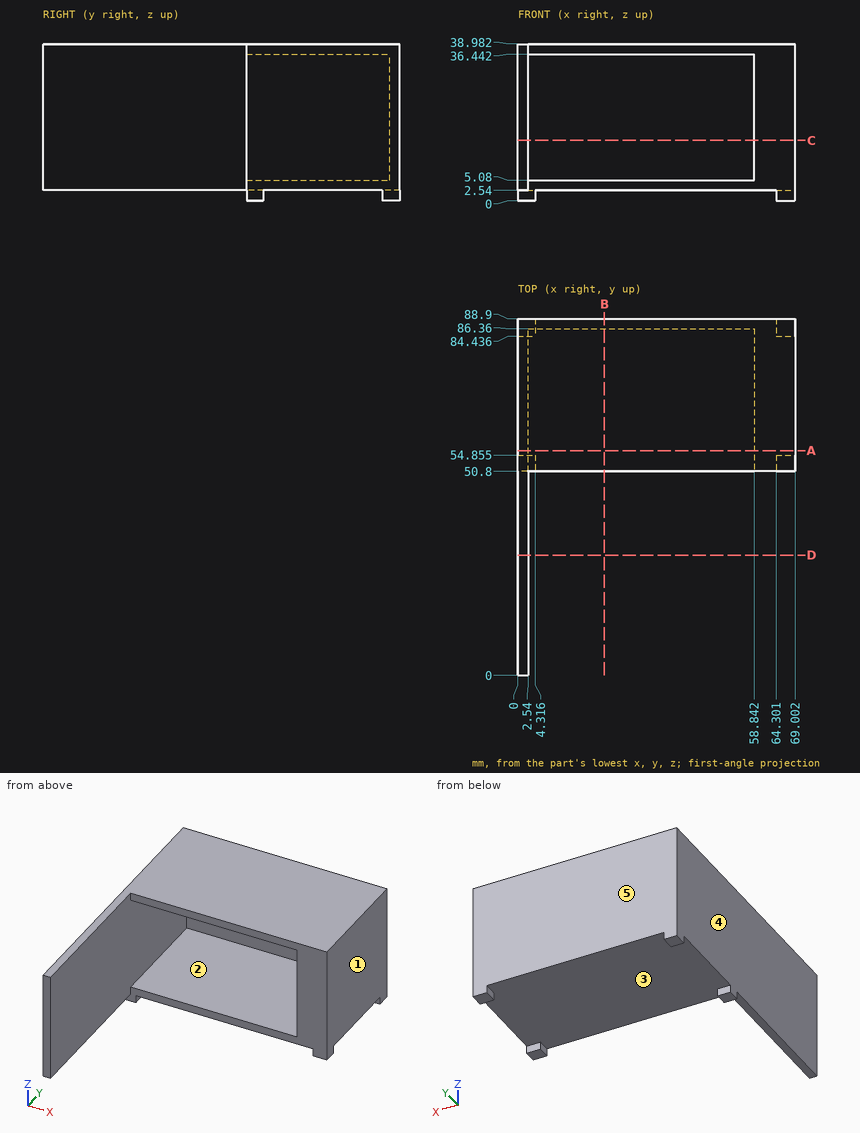
Study the drawing (mm; zero at the part's minimum x, y, z) and answer. A direction names the side the tool comes from. Coordinates: 2 decimals unless noted, no trailing zeros. Write each loop counter-clockwise with the first axis right and the second up, starting at its lowest first coordinate (ties: lowest second). Pieces come first, ordered by that corner, then holes. Notation, with made-up numbers: (12, 58) - (60, 58) arc R30 cw to (60, 81) - close; hole circle Ø1 at (48, 24). An arc over 180 degrees is marked (long way). Answer as a JSON object with one key per item and string values.
Q1. Find section B-B (x = 21.5). Write down the section's boundary in (y, z), plus the area to 3 significant figures.
Results list:
{"outline": "(50.8, 2.54) - (88.9, 2.54) - (88.9, 38.98) - (50.8, 38.98) - (50.8, 36.44) - (86.36, 36.44) - (86.36, 5.08) - (50.8, 5.08) - close", "area": "273 mm^2"}
Q2. Given pin 1 Ø18 at (x, y) = (39, 73.5) entering from -Z; pin 2 Ø5 at (y, z) = (13, 12.5) entering from +X; pin 3 Ø0.8 at (x, z) = (2.5, 1) entering from -Y, each flat-ended and moving along its own axis, determine where each tip first touches the part or whether it passes through.
Results list:
{"pin 1": "stops at z = 2.54", "pin 2": "stops at x = 2.54", "pin 3": "stops at y = 50.8"}
Q3. Consider L1, parallel to X at y = 57.5, z = 13.5; L2, parallel to Z at x = 46.5, y = 66; L3, parallel to Z at x = 63.5, y = 58. Determine where each line is inside the solid, lowest interval first. Write a range as from..to.
Results list:
{"L1": "x = 0..2.54, 58.84..69", "L2": "z = 2.54..5.08, 36.44..38.98", "L3": "z = 2.54..38.98"}
Q4. Find section A-A (y = 56). Write down the section's boundary in (x, z), plus the area to 3 significant figures.
Results list:
{"outline": "(0, 2.54) - (69, 2.54) - (69, 38.98) - (0, 38.98) - close; hole (2.54, 5.08) - (58.84, 5.08) - (58.84, 36.44) - (2.54, 36.44) - close", "area": "749 mm^2"}
Q5. Find section D-D (y = 30). Write down the section's boundary in (x, z).
Results list:
{"outline": "(0, 2.54) - (2.54, 2.54) - (2.54, 38.98) - (0, 38.98) - close"}
Q6. Which of the six approach directions +Z, -Z, +X, -X, +Y, -Y give full straight-line access (tool end or side, diameter ignored) to the marked faces 1 and 2?
Results list:
{"face 1": "+Z, -Z, +X, +Y, -Y", "face 2": "-Y"}
Q7. For a pull along Y with two mould halves and no side action, classify the marked faces 3, 4 and 5 as pulls with the +Y half, pulls with the -Y half, needs draft (parallel to the pull), parting line crosses it, or undercut.
Results list:
{"face 3": "undercut", "face 4": "needs draft", "face 5": "pulls with the +Y half"}
Q8. Find section C-C (z = 15). Write down the section's boundary in (x, y).
Results list:
{"outline": "(0, 0) - (2.54, 0) - (2.54, 86.36) - (58.84, 86.36) - (58.84, 50.8) - (69, 50.8) - (69, 88.9) - (0, 88.9) - close"}
